Autodesk Inventor part; units mm, degrees
ref_plane "Arbeitsebene1" through (14.88, 0, 0) normal (1, 0, 0) x (0, 1, 0)
ref_plane "XZ Plane" through (0, 0, 0) normal (0, 1, 0) x (-1, 0, 0)
ref_plane "XY Plane" through (0, 0, 0) normal (0, 0, 1) x (1, 0, 0)
sketch "Skizze1" plane through (0, 0, 0) normal (0, 0, 1) x (1, 0, 0)
  line L0 (-68.1013, 0) -> (71.8987, 0)
  line L1 (0, -64.8603) -> (0, 47.8406)
  line L2 (-48.1013, 31.7405) -> (51.8987, 31.7405)
  line L3 (51.8987, 31.7405) -> (51.8987, -48.2595)
  line L4 (51.8987, -48.2595) -> (-48.1013, -48.2595)
  line L5 (-48.1013, -48.2595) -> (-48.1013, 31.7405)
  point P0 (0, 0)
  dimension "d0" = 100
  dimension "d1" = 80
extrude "Extrusion1" add sketch "Skizze1" along normal blind 20
fillet "Rundung1" radius 2 4 edges at (1.8987, 31.7405, 20) (-48.1013, -8.2595, 20) (51.8987, -8.2595, 20) (1.8987, -48.2595, 20)
fillet "Rundung2" radius 2 12 edges at (51.8987, -8.2595, 0) (1.8987, 31.7405, 0) (1.8987, -48.2595, 0) (-48.1013, -8.2595, 0) (51.3129, 31.1547, 19.4142) (51.8987, 31.7405, 9) (-47.5155, 31.1547, 19.4142) (-48.1013, 31.7405, 9) (51.3129, -47.6737, 19.4142) (51.8987, -48.2595, 9) (-47.5155, -47.6737, 19.4142) (-48.1013, -48.2595, 9)
sketch "Skizze2" plane through (0, 0, 0) normal (0, 0, -1) x (-1, 0, 0)
  line L0 (16.1013, 1.7405) -> (16.1013, -18.2595)
  line L1 (-19.8987, -18.2595) -> (-19.8987, 1.7405)
  line L2 (-49.8987, 29.7405) -> (46.1013, 29.7405)
  line L3 (-49.8987, -46.2595) -> (-49.8987, 29.7405)
  line L4 (46.1013, 29.7405) -> (46.1013, -46.2595)
  line L5 (-14.8987, -18.2595) -> (-14.8987, 1.7405)
  line L6 (11.1013, -18.2595) -> (11.1013, 1.7405)
  line L7 (-19.8987, 1.7405) -> (-14.8987, 1.7405)
  line L8 (11.1013, 1.7405) -> (16.1013, 1.7405)
  line L9 (16.1013, -18.2595) -> (11.1013, -18.2595)
  line L10 (-14.8987, -18.2595) -> (-19.8987, -18.2595)
  point P0 (0, 0)
  dimension "d8" = 30
  dimension "d9" = 30
  dimension "d10" = 5
  dimension "d11" = 5
  dimension "d12" = 20
  dimension "d13" = 20
extrude "Extrusion2" add sketch "Skizze2" along normal blind 20
fillet "Rundung3" radius 5 4 edges at (17.3987, 1.7405, -20) (17.3987, -18.2595, -20) (-13.6013, 1.7405, -20) (-13.6013, -18.2595, -20)
sketch "Skizze3" plane through (0, 0, 20) normal (0, 0, 1) x (1, 0, 0)
  point P0 (0, 0)
sketch "Skizze4" plane through (19.8987, -18.2595, 0) normal (1, 0, 0) x (0, 0, -1)
  line L0 (0, 0) -> (15, 0)
  line L1 (20, 15) -> (20, 5)
  circle A0 centre (10, 10) radius 2.5
  point P0 (0, 18.2595)
  dimension "d17" = 10
  dimension "d18" = 10
  dimension "d19" = 5
extrude "Extrusion3" cut sketch "Skizze4" against normal blind 40
sketch "Skizze5" plane through (19.8987, -18.2595, 0) normal (1, 0, 0) x (0, 0, -1)
  point P0 (0, 18.2595)
ref_plane "Arbeitsebene1" through (14.88, 0, 0) normal (1, 0, 0) x (0, 1, 0)
sketch "Skizze6" plane through (14.88, 0, 0) normal (1, 0, 0) x (0, 1, 0)
  line L0 (-7.91, 0.6008) -> (-48.7601, -37.6418)
  line L1 (-48.7601, -58.1892) -> (2.3413, -10.3495)
  line L2 (2.3413, -10.3495) -> (-7.91, 0.6008)
  circle A0 centre (-8.2595, -10) radius 2.5
  line L3 (-48.7601, -58.1892) -> (-48.7601, -37.6418)
  point P0 (0, 0)
  dimension "d23" = 7.5
  dimension "d24" = 7.5
  dimension "d25" = 15
  dimension "d26" = 70
  dimension "d27" = 46.888
extrude "Extrusion4" add sketch "Skizze6" against normal blind 25.98 contours L2 L1 L3 L0 | A0
fillet "Rundung4" radius 5 1 edges at (1.89, 2.3413, -10.3495)
sketch "Skizze7" plane through (-11.1, 0, 0) normal (-1, 0, 0) x (0, 0, 1)
  circle A0 centre (-10, -8.2595) radius 2.5
  circle A1 centre (-10, -8.2595) radius 2.5
  point P0 (0, 0)
  point P1 (-10.0246, -8.2595)
  dimension "d31" = 0
extrude "Extrusion5" add sketch "Skizze7" along normal blind 5
sketch "Skizze8" plane through (14.88, 0, 0) normal (1, 0, 0) x (0, 0, -1)
  circle A0 centre (10, -8.2595) radius 2.5
  circle A1 centre (10, -8.2595) radius 2.5
  point P0 (0, 0)
  point P1 (9.9522, -8.2595)
  dimension "d34" = 0
extrude "Extrusion6" add sketch "Skizze8" along normal blind 5
properties part number "Lampe"
Input: part model. Units: mm. Frame: model coordinates. A direction names the side the tool comes from. Give positions to 0.01 mm unless a question says otherwise; leave off trailing zeros. Loops run counter-clockwise (first coordinate to the right, second up) from the corner with the lowest first, then second, coordinate; pieces in that order, holes last. Notation, with made-up numbers: (73.25, 75.25) -> (126.25, 75.25) arc R18 ccw to (126.25, 93.25) -> close; hole circle Ø7 at (43.25, -16). An arc over 180 degrees is marked (long way). Use a Markdown table: item, result.
Q1. Section query C-C, the plane y = 19. Return the cut outline in (x, z).
Entries:
| item | result |
|---|---|
| outline | (-48.1, 2) arc R2 ccw to (-46.1, 0) -> (49.9, 0) arc R2 ccw to (51.9, 2) -> (51.9, 18) arc R2 ccw to (49.9, 20) -> (-46.1, 20) arc R2 ccw to (-48.1, 18) -> close |
Q2. Section query D-D, the plane y = -40.5. Return the cut outline in (x, z), plus the area to 3 significant figures.
Entries:
| item | result |
|---|---|
| outline | (-48.1, 2) arc R2 ccw to (-46.1, 0) -> (49.9, 0) arc R2 ccw to (51.9, 2) -> (51.9, 18) arc R2 ccw to (49.9, 20) -> (-46.1, 20) arc R2 ccw to (-48.1, 18) -> close; (-11.1, -50.46) -> (14.88, -50.46) -> (14.88, -29.91) -> (-11.1, -29.91) -> close |
| area | 2,530 mm² |
Q3. First-contact query: P1, Ø2.5, axis at x = 16, y = -7, coming from the -Z side; P2, Ø6, axis at y = -8.26, z = -10, coming from the +X side; P3, Ø6.5, axis at y = -8.26, z = -10, coming from the -X side. Flat tips, straight axial feed; report the tip coordinate or a pass-through.
Entries:
| item | result |
|---|---|
| P1 | stops at z = -20 |
| P2 | stops at x = 19.9 |
| P3 | stops at x = -16.1 |
Q4. Pull-direction query (Y, two-part tool) for faces 1 (the flat face through (1, 1, 0)), 2 (the cylindrical face through (17.43, -16.83, -18.5)), 3 (the flat face through (-11.1, -26, -29)); classes: pulls with the +Y half, pulls with the -Y half, needs draft (parallel to the pull), parting line crosses it, or undercut.
Entries:
| item | result |
|---|---|
| face 1 | needs draft |
| face 2 | pulls with the -Y half |
| face 3 | undercut |
Q5. Access query for faces 4 (the cylindrical face through (1.708, 0.273, -10.226)), 5 (the flat face through (19.899, -11, -8)), 6 (the flat face through (-14, 1.74, -7)). Directions: +Z, -Z, +X, -X, +Y, -Y. A direction counts if a zero-diameter tool reaches every point of the face in a straight line with its end or side. Return the directions, or none.
Entries:
| item | result |
|---|---|
| face 4 | +Y |
| face 5 | -Z, +X, +Y, -Y |
| face 6 | -Z, +X, -X, +Y |
Q6. Section query A-A, the plane x = 0. Return the cut outline in (y, z), plus the area to 3 significant figures.
Entries:
| item | result |
|---|---|
| outline | (-48.76, -58.19) -> (-1.31, -13.77) arc R5 ccw to (-1.08, -6.7) -> (-7.35, 0) -> (29.74, 0) arc R2 ccw to (31.74, 2) -> (31.74, 18) arc R2 ccw to (29.74, 20) -> (-46.26, 20) arc R2 ccw to (-48.26, 18) -> (-48.26, 2) arc R2 ccw to (-46.26, 0) -> (-8.55, 0) -> (-48.76, -37.64) -> close |
| area | 2,540 mm² |
Q7. Section query B-B, the plane z = -5. Return the cut outline in (x, y).
Entries:
| item | result |
|---|---|
| outline | (-16.1, -18.26) -> (-11.1, -18.26) -> (-11.1, 1.74) -> (-16.1, 1.74) -> close; (-11.1, -13.89) -> (14.88, -13.89) -> (14.88, -2.67) -> (-11.1, -2.67) -> close; (14.9, -18.26) -> (19.9, -18.26) -> (19.9, 1.74) -> (14.9, 1.74) -> close |
Q8. Ray query, probe 1 along Z at (x, y) = (-10, 21.5); probe 2 along X at (y, z) = (-16.5, -25); probe 3 along Z at (x, y) = (7.5, -18.5). Return the intervals inside material, ascending. Write a range as from..to.
Entries:
| item | result |
|---|---|
| probe 1 | z = 0..20 |
| probe 2 | x = -11.1..14.88 |
| probe 3 | z = -29.86..-9.31, 0..20 |
